from build123d import *

# Parameters (mm, degrees)
BOX014_W          = 3
BOX014_H          = 3
BOX014_DEPTH      = 8
BOX013_W          = 3
BOX013_H          = 3
BOX013_DEPTH      = 8
CYLINDER009_R     = 3.5
CYLINDER009_DEPTH = 25


with BuildPart() as pivotrodbodypinhole4:
    # Box014 → Box014 (new body)
    with BuildSketch(Plane(origin=(18, 62, 10), x_dir=(1, 0, 0), z_dir=(0, 0, 1))):
        with Locations((1.5, 1.5)):
            Rectangle(BOX014_W, BOX014_H)
    extrude(amount=BOX014_DEPTH)


with BuildPart() as pivotrodpinholesright:
    # Box013 → Box013 (new body)
    with BuildSketch(Plane(origin=(18, 79, 10), x_dir=(1, 0, 0), z_dir=(0, 0, 1))):
        with Locations((1.5, 1.5)):
            Rectangle(BOX013_W, BOX013_H)
    extrude(amount=BOX013_DEPTH)

    # Fusion009: union PivotRodBodyPinhole4
    add(pivotrodbodypinhole4.part)


with BuildPart() as pivotrodright:
    # Cylinder009 → Cylinder009 (new body)
    with BuildSketch(Plane(origin=(19.5, 84.5, 14), x_dir=(1, 0, 0), z_dir=(0, -1, 0))):
        Circle(CYLINDER009_R)
    extrude(amount=CYLINDER009_DEPTH)

    # Cut007: cut PivotRodPinholesRight
    add(pivotrodpinholesright.part, mode=Mode.SUBTRACT)


solid = pivotrodright.part
For this review, take the finished solid that the model builds, in its own axes (mm). A direction names the side the tool comes from. Round coordinates to 2 decimals unless told otherwise and drop trailing zeros. Write each loop counter-clockwise with the first axis right and the second up, starting at its lowest first coordinate (ties: lowest second). Pieces come first, ordered by that corner, then holes. Notation, with made-up numbers: (17.25, 88) - (30.25, 88) arc R16 cw to (30.25, 103) - close; hole circle Ø10 at (-39, -5.5). An arc over 180 degrees is marked (long way). Write item = value, one per line. Start each with the question number.
1. Draft analysis for pull direction X (two halves, no side actions). For faces 1 (the face through (19, 59.5, 14)), 2 (the face through (22.733, 72.175, 12.659)), 3 (the face through (18, 63, 14)), state which applies: released by +X, released by -X, zero draft, split by the parting line, or undercut.
2. Consider section C-C on y = 64.5. State the section outline as (x, z) points, plus the area to 3 significant figures.
3. Consider section A-A on x = 19.5. State the section outline as (y, z) points.
4. For faces 4 (the face through (19, 84.5, 14)), 5 (the face through (21, 80, 14)), list the 3-axis set-ups (+Z, -Z, +X, -X, +Y, -Y) from which the entire face can be reached by the end or side of a thin tool; tool diameter is ignored.
5. For pin 1 Ø0.9 at (y, z) = (80.5, 13.5) entering from +X, flat-tipped, find the tip position at first contact; note if it passes through.
6. Consider section D-D on z = 12.25. State the section outline as (x, y) points.
7. Consider section B-B on z = 14. State the section outline as (x, y) points, plus the area to 3 significant figures.
8. Wall thickness on L1, parallel to Y at x = 18.5, z = 11; L2, parallel to X at y = 79.75, z = 11.5; L3, parallel to Z at x = 21.75, y = 61.75: over which ranges is each line inside the solid? List them lowest first.
Evaluation:
q1.face_1 = zero draft
q1.face_2 = split by the parting line
q1.face_3 = undercut
q2.outline = (18, 10.84) - (18, 17.16) arc R3.5 ccw to start; (21, 10.84) arc R3.5 ccw to (21, 17.16) - close
q2.area = 18.1 mm2
q3.outline = (59.5, 10.5) - (62, 10.5) - (62, 17.5) - (59.5, 17.5) - close; (65, 10.5) - (79, 10.5) - (79, 17.5) - (65, 17.5) - close; (82, 10.5) - (84.5, 10.5) - (84.5, 17.5) - (82, 17.5) - close
q4.face_4 = +Z, -Z, +X, -X, +Y
q4.face_5 = +Z, -Z
q5.pin_1 = 23
q6.outline = (16.47, 59.5) - (22.53, 59.5) - (22.53, 84.5) - (16.47, 84.5) - close; hole (18, 62) - (21, 62) - (21, 65) - (18, 65) - close; hole (18, 79) - (21, 79) - (21, 82) - (18, 82) - close
q7.outline = (16, 59.5) - (23, 59.5) - (23, 84.5) - (16, 84.5) - close; hole (18, 62) - (21, 62) - (21, 65) - (18, 65) - close; hole (18, 79) - (21, 79) - (21, 82) - (18, 82) - close
q7.area = 157 mm2
q8.L1 = 59.5 to 62, 65 to 79, 82 to 84.5
q8.L2 = 17.05 to 18, 21 to 21.95
q8.L3 = 11.32 to 16.68
